Read the model definition and answer for the solid it produces. Units are mm, in the model's axes. Give positions to 0.01 mm unless a question says otherwise; leave off trailing zeros. Order: outer loops, then holes, each group sorted by start corner. A loop starts at its lowest first (then second) coordinate and runs counter-clockwise, first axis right, second up.
Item 1: Given pin 1 Ø1 at (x, z) = (4.5, 70.5) entering from -Y; pin 2 Ø1.5 at (x, z) = (-3, 84) entering from -Y; pin 3 Ø4 at (x, z) = (-1, 37.5) entering from -Y, each flat-ended and moving along its own axis, determine where each tip first touches the part or whether it passes through.
Item 2: A cutting plane is placed at B-B (x = -2.75). Write down the section's boundary in (y, z), plus the area to 3 significant figures.
Item 3: Find the intervals of material crossed by line 1 along Y through (x, z) = (-4.75, 152); line 2 along X through (y, z) = (-6.5, 165.5); line 3 along X through (y, z) = (5.75, 170.5), in increasing order.
Item 4: A cutting plane is placed at A-A (z = 40). Write down the section's boundary in (x, y).
from build123d import *

# Parameters (mm, degrees)
F1_DEPTH = 195
F2_SIZE  = 1.5


with BuildPart() as f1:
    # F0 (on Top) → F1 (new body)
    with BuildSketch(Plane.XY):
        Polygon((7, -4.041452), (7, 4.041452), (0, 8.082904), (-7, 4.041452), (-7, -4.041452), (0, -8.082904), align=None)
    extrude(amount=F1_DEPTH)

    # F2
    f2_edges = [f1.edges().sort_by_distance(p)[0] for p in [
        (-3.5, -6.062178, 195),
        (3.5, -6.062178, 195),
        (7, 0, 195),
        (3.5, 6.062178, 195),
        (-3.5, 6.062178, 195),
        (-7, 0, 195),
    ]]
    chamfer(f2_edges, length=F2_SIZE)


solid = f1.part
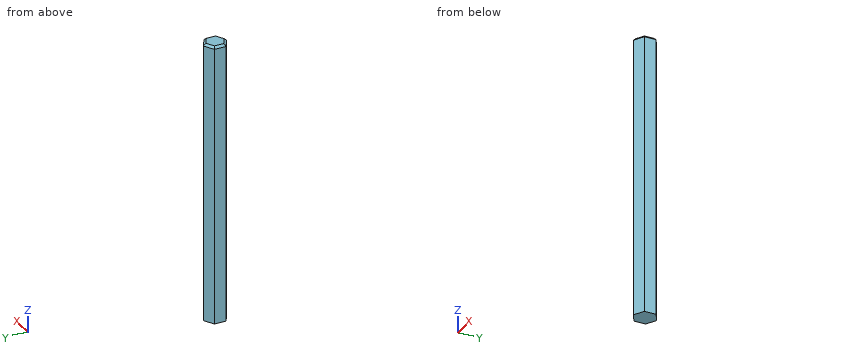
Response values:
1. pin 1: stops at y = -5.77
1. pin 2: stops at y = -6.78
1. pin 3: stops at y = -8.08
2. outline: (-6.5, 0) - (6.5, 0) - (6.5, 193.5) - (4.76, 195) - (-4.76, 195) - (-6.5, 193.5) - close
2. area: 2,530 mm2
3. line 1: y = -5.34 to 5.34
3. line 2: x = -2.74 to 2.74
3. line 3: x = -4.04 to 4.04
4. outline: (-7, -4.04) - (0, -8.08) - (7, -4.04) - (7, 4.04) - (0, 8.08) - (-7, 4.04) - close
